from build123d import *

# Parameters (mm, degrees)
EXTRUDE_THIN1_DEPTH = 24
SKETCH2_R           = 1.5
CUT_EXTRUDE1_DEPTH  = 10
SKETCH3_R           = 1.5
CUT_EXTRUDE2_DEPTH  = 10
FILLET1_R           = 1
FILLET2_R           = 0.5
FILLET3_R           = 0.5
SKETCH4_R           = 5
CUT_EXTRUDE3_DEPTH  = 10
CUT_EXTRUDE5_DEPTH  = 10


with BuildPart() as part:
    # Sketch1 → Extrude-Thin1 (new body)
    with BuildSketch(Plane.XY):
        Polygon((-6.621018809, 22), (0, 22), (0, 0), (14, 0), (14, -0.5), (-0.5, -0.5), (-0.5, 21.5), (-6.621018809, 21.5), align=None)
    extrude(amount=EXTRUDE_THIN1_DEPTH)

    # Sketch2 → Cut-Extrude1 (cut)
    with BuildSketch(Plane(origin=(0, 0, 0), x_dir=(1, 0, 0), z_dir=(0, 1, 0))):
        with Locations(Location((10, -19, 0), (0, 0, 270))):
            Circle(SKETCH2_R)
        with Locations(Location((10, -9, 0), (0, 0, 270))):
            Circle(SKETCH2_R)
    extrude(amount=-CUT_EXTRUDE1_DEPTH, mode=Mode.SUBTRACT)

    # Sketch3 → Cut-Extrude2 (cut)
    with BuildSketch(Plane(origin=(0, 0, 0), x_dir=(0, 0, -1), z_dir=(1, 0, 0))):
        with Locations((-16.7, 19.2)):
            Circle(SKETCH3_R)
        with Locations((-16.7, 2.5)):
            Circle(SKETCH3_R)
        with Locations((-6.7, 19.2)):
            Circle(SKETCH3_R)
        with Locations((-6.7, 2.5)):
            Circle(SKETCH3_R)
    extrude(amount=-CUT_EXTRUDE2_DEPTH, mode=Mode.SUBTRACT)

    # Fillet1
    fillet1_edges = [part.edges().sort_by_distance(p)[0] for p in [
        (14, -0.25, 24),
    ]]
    fillet(fillet1_edges, radius=FILLET1_R)

    # Fillet2
    fillet2_edges = [part.edges().sort_by_distance(p)[0] for p in [
        (-0.5, -0.5, 12),
        (-0.5, 21.5, 12),
        (0, 0, 12),
        (-6.621018809, 21.75, 24),
        (-6.621018809, 21.75, 0),
        (14, -0.25, 0),
    ]]
    fillet(fillet2_edges, radius=FILLET2_R)

    # Fillet3
    fillet3_edges = [part.edges().sort_by_distance(p)[0] for p in [
        (0, 22, 12),
    ]]
    fillet(fillet3_edges, radius=FILLET3_R)

    # Sketch4 → Cut-Extrude3 (cut)
    with BuildSketch(Plane(origin=(0, 0, 0), x_dir=(0, 0, -1), z_dir=(1, 0, 0))):
        with Locations(Location((-12, 10.5, 0), (0, 0, 90))):
            Circle(SKETCH4_R)
    extrude(amount=-CUT_EXTRUDE3_DEPTH, mode=Mode.SUBTRACT)

    # Sketch5 → Cut-Extrude5 (cut)
    with BuildSketch(Plane(origin=(0, 0, 0), x_dir=(0, 0, -1), z_dir=(1, 0, 0))):
        with BuildLine():
            Line((0, 15), (0, 7))
            ThreePointArc((0, 7), (-4, 11), (0, 15))
        make_face()
        with BuildLine():
            Line((-24, 14), (-24, 6))
            ThreePointArc((-24, 6), (-20, 10), (-24, 14))
        make_face()
    extrude(amount=-CUT_EXTRUDE5_DEPTH, mode=Mode.SUBTRACT)


solid = part.part
Can you work these out from the model? Positions are in its coordinate system, mm. A direction names the side the tool comes from. Coordinates: 2 decimals unless noted, no trailing zeros. Write each loop counter-clockwise with the first axis right and the second up, starting at its lowest first coordinate (ties: lowest second). Pieces come first, ordered by that corner, then holes. Notation, with made-up numbers: (58.5, -19) -> (105.5, -19) arc R16 ccw to (105.5, 1) -> close; hole circle Ø6 at (41.25, -1.5). An arc over 180 degrees is marked (long way). Write each question's results on one line, items separated by ' | '. Start each with the question number.
Item 1: Please list where these lines run through material, in increasing order: probe 1 along Y at (x, z) = (-0.25, 6.7); probe 2 along Y at (x, z) = (-0.3, 6.7); probe 3 along X at (y, z) = (17.5, 22.5).
Item 2: Thinking about a two-plate mould opening in Z: for faces 4 (the cylindrical face through (-0.2, 10.9, 4)), 5 (the flat face through (-4, 22, 12)), 6 (the cylindrical face through (13.699, -0.254, 23.715)), 7 (the cylindrical face through (9.1, -0.2, 7.8)), which applies, released by +Z, released by -Z, zero draft, split by the parting line, or undercut?
Item 3: I'm going to push flat-ended pins straight in: P1, Ø6.5, axis at y = 14.5, z = 12.5, coming from the -X side; P2, Ø4, axis at x = 10.5, z = 8, coming from the +Y side; P3, Ø5, axis at x = -1, y = 7, coming from the -Z side; P4, Ø6, axis at y = 18.5, z = 11.5, coming from the +X side. Where does each tip first touch, or does it pass through?
Item 4: If we section it at D-D, the plane z = 19: Write out the boundary of the cut face in (x, y).
Item 5: If we section it at B-B, the plane z = 9: Write out the boundary of the cut face in (x, y).
Item 6: On a 3-axis mill with a long thin cutter (end or side, diameter ignored), from which of +Z, -Z, +X, -X, +Y, -Y can I reach the whole of each face in a straight line? I mean faces 1 (the flat face through (0, 16, 12)), 2 (the flat face through (-4, 21.5, 12)), 3 (the flat face through (-0.3, 20.1, 0)). Say none if no direction works.
Item 7: If we section it at C-C, the plane x = 10: Write out the boundary of the cut face in (y, z).
Item 8: If we section it at A-A, the plane y = 19.2: Write out the boundary of the cut face in (x, z), and give its area (3 significant figures).
Answer block:
1) probe 1: -0.43 to 1, 4 to 17.7, 20.7 to 21.93 | probe 2: -0.4 to 1, 4 to 17.7, 20.7 to 21.96 | probe 3: -0.5 to 0
2) face 4: released by -Z | face 5: zero draft | face 6: released by +Z | face 7: undercut
3) P1: x = -0.5 | P2: y = 0 | P3: z = 0 | P4: x = 0
4) outline: (-6.62, 21.5) -> (-1, 21.5) arc R0.5 cw to (-0.5, 21) -> (-0.5, 0) arc R0.5 ccw to (0, -0.5) -> (8.5, -0.5) -> (8.5, 0) -> (0.5, 0) arc R0.5 cw to (0, 0.5) -> (0, 21.5) arc R0.5 ccw to (-0.5, 22) -> (-6.62, 22) -> close; (11.5, -0.5) -> (14, -0.5) -> (14, 0) -> (11.5, 0) -> close
5) outline: (-6.62, 21.5) -> (-1, 21.5) arc R0.5 cw to (-0.5, 21) -> (-0.5, 14.5) -> (0, 14.5) -> (0, 21.5) arc R0.5 ccw to (-0.5, 22) -> (-6.62, 22) -> close; (-0.5, 0) arc R0.5 ccw to (0, -0.5) -> (8.5, -0.5) -> (8.5, 0) -> (0.5, 0) arc R0.5 cw to (0, 0.5) -> (0, 6.5) -> (-0.5, 6.5) -> close; (11.5, -0.5) -> (14, -0.5) -> (14, 0) -> (11.5, 0) -> close
6) face 1: +Z, -Z, +X, +Y | face 2: +Z, -Z, -X, -Y | face 3: -Z, +X, -X, +Y, -Y
7) outline: (-0.5, 0) -> (0, 0) -> (0, 7.5) -> (-0.5, 7.5) -> close; (-0.5, 10.5) -> (0, 10.5) -> (0, 17.5) -> (-0.5, 17.5) -> close; (-0.5, 20.5) -> (0, 20.5) -> (0, 24) -> (-0.5, 24) -> close
8) outline: (-0.5, 0) -> (0, 0) -> (0, 5.2) -> (-0.5, 5.2) -> close; (-0.5, 8.2) -> (0, 8.2) -> (0, 15.2) -> (-0.5, 15.2) -> close; (-0.5, 18.2) -> (0, 18.2) -> (0, 24) -> (-0.5, 24) -> close | area: 9.00 mm²
